from build123d import *

# Parameters (mm, degrees)
F1_DEPTH      = 2
F0_R          = 2.75
F2_DEPTH      = 7.5
F4_R          = 3.3
F5_DEPTH      = 1
F5_DEPTH_BACK = 2
F7_DEPTH      = 2
F8_W          = 6.7
F8_H          = 6.7
F8_R          = 3.3
F9_DEPTH      = 1


# Not quite as in the source:
# - after a boolean that leaves OpenCascade's solid faulty, fix() repairs it


with BuildPart() as f1:
    # F0 (on Top) → F1 (new body)
    with BuildSketch(Plane.XY):
        with BuildLine():
            ThreePointArc((20.6, 10.25), (12.4912427894, 6.8912427894), (15.85, 15))
            Line((15.85, 15), (-15.85, 15))
            ThreePointArc((-15.85, 15), (-12.4912427894, 13.6087572106), (-11.1, 10.25))
            ThreePointArc((-11.1, 10.25), (-15.85, 5.5), (-20.6, 10.25))
            Line((-20.6, 10.25), (-20.6, -12))
            ThreePointArc((-20.6, -12), (-19.7213203436, -14.1213203436), (-17.6, -15))
            Line((-17.6, -15), (17.6, -15))
            ThreePointArc((17.6, -15), (19.7213203436, -14.1213203436), (20.6, -12))
            Line((20.6, -12), (20.6, 10.25))
        make_face()
    extrude(amount=F1_DEPTH)

    # F0 (on Top) → F2 (join, symmetric)
    with BuildSketch(Plane.XY):
        with BuildLine():
            ThreePointArc((-11.1, 10.25), (-12.4912427894, 13.6087572106), (-15.85, 15))
            ThreePointArc((-15.85, 15), (-19.2087572106, 13.6087572106), (-20.6, 10.25))
            ThreePointArc((-20.6, 10.25), (-15.85, 5.5), (-11.1, 10.25))
        make_face()
        with Locations((-15.85, 10.25)):
            Circle(F0_R, mode=Mode.SUBTRACT)
        with BuildLine():
            ThreePointArc((20.6, 10.25), (19.2087572106, 13.6087572106), (15.85, 15))
            ThreePointArc((15.85, 15), (12.4912427894, 6.8912427894), (20.6, 10.25))
        make_face()
        with Locations((15.85, 10.25)):
            Circle(F0_R, mode=Mode.SUBTRACT)
    extrude(amount=F2_DEPTH, both=True)

    # F4 (on line) → F5 (join, two sides)
    with BuildSketch(Plane(origin=(0, 10.25, 0), x_dir=(-1, 0, 0), z_dir=(0, 1, 0))) as f5_sk:
        with BuildLine():
            Line((-13.1, 7.5), (-13.1, 2))
            Line((-13.1, 2), (-11.1, 2))
            Line((-11.1, 2), (11.1, 2))
            Line((11.1, 2), (13.1, 2))
            Line((13.1, 2), (13.1, 7.5))
            Line((13.1, 7.5), (11.1, 7.5))
            ThreePointArc((11.1, 7.5), (10.5142135624, 8.9142135624), (9.1, 9.5))
            Line((9.1, 9.5), (-9.1, 9.5))
            ThreePointArc((-9.1, 9.5), (-10.5142135624, 8.9142135624), (-11.1, 7.5))
            Line((-11.1, 7.5), (-13.1, 7.5))
        make_face()
        with Locations((-5.1, 5.5)):
            Circle(F4_R, mode=Mode.SUBTRACT)
    extrude(amount=F5_DEPTH)
    extrude(f5_sk.sketch, amount=-F5_DEPTH_BACK)

    # F6 (on face) → F7 (cut, through all)
    with BuildSketch(Plane.XY.offset(2)):
        with BuildLine():
            ThreePointArc((-15.85, 15), (-12.8656659034, 13.9454363748), (-11.2064560947, 11.25))
            Line((-11.2064560947, 11.25), (11.2064560947, 11.25))
            ThreePointArc((11.2064560947, 11.25), (12.8656659034, 13.9454363748), (15.85, 15))
            Line((15.85, 15), (-15.85, 15))
        make_face()
    extrude(amount=-F7_DEPTH, mode=Mode.SUBTRACT)

    # F8 (on face) → F9 (cut)
    with BuildSketch(Plane.XZ.offset(-8.25)):
        with Locations((5.1, 5.5)):
            Rectangle(F8_W, F8_H)
        with Locations((5.1, 5.5)):
            Circle(F8_R, mode=Mode.SUBTRACT)
        with Locations((5.1, 5.5)):
            Circle(F8_R)
    extrude(amount=-F9_DEPTH, mode=Mode.SUBTRACT)

    add(f1.part.fix(), mode=Mode.REPLACE)


solid = f1.part
Can you work these out from the model? Positions are in its coordinate system, mm. A direction names the side the tool comes from. Round coordinates to 2 decimals unless told otherwise and drop trailing zeros. Loops run counter-clockwise (first coordinate to the right, second up) from the corner with the lowest first, then second, coordinate; pieces in that order, holes last. Notation, with made-up numbers: (-37.5, 2.25) - (-22.5, 2.25) arc R8 ccw to (-22.5, 12.25) - close; hole circle Ø11 at (-3, 36). An arc over 180 degrees is marked (long way). Write item = value, one per line. Start each with the question number.
(1) For P1, Ø3, axis at x = 9, y = 8, coming from the -Z side; P2, Ø5, axis at x = -14.5, y = 11.5, coming from the +Z side; P3, Ø5, axis at x = 2.5, z = 7, coming from the -Y side, each with a flat end and sliding along its axis, tell me the tip position at first contact or that it passes through.
(2) If we section it at D-D (z = 8.25): Please give me the cut outline in (x, y), and give its area (3 significant figures).
(3) If we section it at A-A (z = 1.5): Please give me the cut outline in (x, y).
(4) If we section it at B-B (x = 5.1): Please give me the cut outline in (y, z).
(5) If we mould it in two halves opening along X, with no side actions, what happens to faces 1 (the face through (-19.74, -14.1, 0.99)), 2 (the face through (10.5, 9.73, 8.93)), 3 (the face through (5.53, 10.24, 8.77))? For each: released by +X, released by -X, zero draft, split by the parting line, or undercut.
(6) If I drill on probe 1 along X at (y, z) = (10.15, 5.5); probe 2 along X at (y, z) = (11.75, -2.25); probe 3 along Y at (x, z) = (-8, 3), over which ranges is the centre line in solid material (lowest first)? Write a range as [from, to].
(7) If we section it at C-C (z = -5): Please give me the cut outline in (x, y), and give its area (3 significant figures).
(8) For faces 4 (the face through (-2, 8.25, 6)), 5 (the face through (-12.7, 10.2, 7.5)), 6 (the face through (8.45, 9, 5)), 7 (the face through (18, 8, 7.5)), which set-ups out of +Z, -Z, +X, -X, +Y, -Y let a thin tool reach every point of the face, with its end or its side?
Ans:
q1.P1 = 0
q1.P2 = 7.5
q1.P3 = 8.25
q2.outline = (-10.95, 8.25) - (1.75, 8.25) - (1.75, 9.25) - (3.28, 9.25) - (3.28, 11.25) - (-10.95, 11.25) - close; (6.92, 9.25) - (8.45, 9.25) - (8.45, 8.25) - (10.95, 8.25) - (10.95, 11.25) - (6.92, 11.25) - close
q2.area = 51.7 mm²
q3.outline = (-20.6, -12) arc R3 ccw to (-17.6, -15) - (17.6, -15) arc R3 ccw to (20.6, -12) - (20.6, 10.25) arc R4.75 ccw to (11.21, 11.25) - (-11.21, 11.25) arc R4.75 ccw to (-20.6, 10.25) - close; hole circle Ø5.5 at (-15.85, 10.25); hole circle Ø5.5 at (15.85, 10.25)
q4.outline = (-15, 0) - (11.25, 0) - (11.25, 2.2) - (9.25, 2.2) - (9.25, 2.15) - (8.25, 2.15) - (8.25, 2) - (-15, 2) - close; (8.25, 8.85) - (9.25, 8.85) - (9.25, 8.8) - (11.25, 8.8) - (11.25, 9.5) - (8.25, 9.5) - close
q5.face_1 = released by -X
q5.face_2 = released by +X
q5.face_3 = undercut
q6.probe_1 = [-20.6, -18.6], [-13.1, 1.8], [8.4, 13.1], [18.6, 20.6]
q6.probe_2 = [-20.36, -18.15], [-13.55, -11.34], [11.34, 13.55], [18.15, 20.36]
q6.probe_3 = [8.25, 11.25]
q7.outline = circle Ø9.5 at (-15.85, 10.25); circle Ø9.5 at (15.85, 10.25); hole circle Ø5.5 at (-15.85, 10.25); hole circle Ø5.5 at (15.85, 10.25)
q7.area = 94.2 mm²
q8.face_4 = +Z, -Y
q8.face_5 = +Z, -X, +Y, -Y
q8.face_6 = -Y
q8.face_7 = +Z, +X, +Y, -Y
